```python
from build123d import *

# Parameters (mm, degrees)
SKETCH_1_W          = 42
SKETCH_1_H          = 42
EXTRUDE_1_DEPTH     = 54
EXTRUDE_START       = 54
EXTRUDE_2_DEPTH     = 22.5
FILLET_1_R          = 0.5
CUT_EXTRUDE_START   = 54
SKETCH_3_R          = 1.5
CUT_EXTRUDE_1_DEPTH = 10


with BuildPart() as part:
    # 草图1 → 凸台-拉伸1 (new body)
    with BuildSketch(Plane.XY):
        Rectangle(SKETCH_1_W, SKETCH_1_H)
    extrude(amount=EXTRUDE_1_DEPTH)

    # 草图2 → 凸台-拉伸2 (add)
    with BuildSketch(Plane.XY.offset(EXTRUDE_START)):
        with BuildLine():
            Line((-1.785837809, -1.749509451), (1.844440663, -1.687613298))
            ThreePointArc((1.844440663, -1.687613298), (-0.042618741, 2.499636702), (-1.785837809, -1.749509451))
        make_face()
    extrude(amount=EXTRUDE_2_DEPTH)

    # 圆角1
    fillet_1_edges = [part.edges().sort_by_distance(p)[0] for p in [
        (-21, 0, 54),
        (0, -21, 54),
        (21, 0, 54),
        (0, -21, 0),
        (-21, 0, 0),
        (0, 21, 0),
        (21, 0, 0),
        (21, -21, 27),
        (-21, -21, 27),
        (-21, 21, 27),
        (21, 21, 27),
        (0, 21, 54),
    ]]
    fillet(fillet_1_edges, radius=FILLET_1_R)

    # 草图3 → 切除-拉伸1 (cut)
    with BuildSketch(Plane.XY.offset(CUT_EXTRUDE_START)):
        with Locations(Location((-15.5, 15.5, 0), (0, 0, 180))):
            Circle(SKETCH_3_R)
        with Locations(Location((15.5, 15.5, 0), (0, 0, 180))):
            Circle(SKETCH_3_R)
        with Locations(Location((15.5, -15.5, 0), (0, 0, 180))):
            Circle(SKETCH_3_R)
        with Locations(Location((-15.5, -15.5, 0), (0, 0, 180))):
            Circle(SKETCH_3_R)
    extrude(amount=-CUT_EXTRUDE_1_DEPTH, mode=Mode.SUBTRACT)


solid = part.part
```
Build history of the part. All positions in model axes, mm. A direction names the side the tool comes from. Give positions to 0.01 mm unless a question says otherwise; leave off trailing zeros. Loops run counter-clockwise (first coordinate to the right, second up) from the corner with the lowest first, then second, coordinate; pieces in that order, holes last. Notation, with made-up numbers: (20.5, 84) -> (30.5, 84) arc R38 ccw to (30.5, 122) -> close; hole circle Ø6 at (-27.75, 51.5). An arc over 180 degrees is marked (long way). One line per question, with ' | ' between items.
Q1. Cut at A-A, the plane z = 45. Write the cut outline in (x, y).
Filled sheet:
outline: (-21, -20.5) arc R0.5 ccw to (-20.5, -21) -> (20.5, -21) arc R0.5 ccw to (21, -20.5) -> (21, 20.5) arc R0.5 ccw to (20.5, 21) -> (-20.5, 21) arc R0.5 ccw to (-21, 20.5) -> close; hole circle Ø3 at (-15.5, -15.5); hole circle Ø3 at (-15.5, 15.5); hole circle Ø3 at (15.5, -15.5); hole circle Ø3 at (15.5, 15.5)
Q2. Drill centre lines: line 1 along X through (y, z) = (-15.5, 50.75); line 2 along X through (y, z) = (15, 46). Where is each one in solid material? Low to high. Write a range as [from, to].
Filled sheet:
line 1: x = [-21, -17], [-14, 14], [17, 21] | line 2: x = [-21, -16.91], [-14.09, 14.09], [16.91, 21]
Q3. Cut at C-C, the plane x = -8. Write the cut outline in (y, z), plus the area to 3 significant figures.
Filled sheet:
outline: (-21, 0.5) arc R0.5 ccw to (-20.5, 0) -> (20.5, 0) arc R0.5 ccw to (21, 0.5) -> (21, 53.5) arc R0.5 ccw to (20.5, 54) -> (-20.5, 54) arc R0.5 ccw to (-21, 53.5) -> close | area: 2,270 mm²
Q4. Drop flat-ended pins along their axis: pin 1 (6 mm diameter, centred on x = 10, y = -1.5, fed in from +Z); pin 2 (0.9 mm diameter, centred on x = 16, y = 15, fed in from +Z). Give the stop position or say it passes through.
Filled sheet:
pin 1: stops at z = 54 | pin 2: stops at z = 44
Q5. Tool access for faces 1 (the flat face through (0, 0, 0)), 2 (the flat face through (16, 15, 44)): list every direction of +Z, -Z, +X, -X, +Y, -Y with a clear straight run to the whole face (end or side of a thin tool).
Filled sheet:
face 1: -Z, +X, -X, +Y, -Y | face 2: +Z
Q6. Cut at B-B, the plane y = -15.5. Write the cut outline in (x, z).
Filled sheet:
outline: (-21, 0.5) arc R0.5 ccw to (-20.5, 0) -> (20.5, 0) arc R0.5 ccw to (21, 0.5) -> (21, 53.5) arc R0.5 ccw to (20.5, 54) -> (17, 54) -> (17, 44) -> (14, 44) -> (14, 54) -> (-14, 54) -> (-14, 44) -> (-17, 44) -> (-17, 54) -> (-20.5, 54) arc R0.5 ccw to (-21, 53.5) -> close
Q7. Pull direction Y, two halves, no side cores. Call faces 3 (the flat face through (-21, 0, 27)), 4 (the cylindrical face through (17, -15.57, 49.07)), 5 (the cylindrical face through (0, 2.5, 65.1)): pulls with the +Y half, pulls with the -Y half, needs draft (parallel to the pull), parting line crosses it, or undercut.
Filled sheet:
face 3: needs draft | face 4: undercut | face 5: parting line crosses it
